from build123d import *

# Parameters (mm, degrees)
BOSS_EXTRUDE1_DEPTH = 534.6
SKETCH2_R           = 12.7
CUT_EXTRUDE1_DEPTH  = 18.288
SKETCH3_R           = 14
CUT_EXTRUDE2_DEPTH  = 18.288
SKETCH4_R           = 14
CUT_EXTRUDE3_DEPTH  = 18.288


with BuildPart() as part:
    # Sketch1 → Boss-Extrude1 (new body)
    with BuildSketch(Plane.XY):
        Polygon((0, 0), (5.762672042, 402.6498479), (18.424747765, 400), (12.7, 0), align=None)
    extrude(amount=BOSS_EXTRUDE1_DEPTH)

    # Sketch2 → Cut-Extrude1 (cut)
    with BuildSketch(Plane(origin=(12.697399197, -0.181723519, 0), x_dir=(0, 0, -1), z_dir=(0.9998976009274501, -0.014310403891230014, 0))):
        with Locations(Location((-88.9, 254.181742129, 0), (0, 0, 90))):
            Circle(SKETCH2_R)
    extrude(amount=-CUT_EXTRUDE1_DEPTH, mode=Mode.SUBTRACT)

    # Sketch3 → Cut-Extrude2 (cut)
    with BuildSketch(Plane(origin=(12.697399197, -0.181723519, 0), x_dir=(0, 0, -1), z_dir=(0.9998976009274501, -0.014310403891230014, 0))):
        with Locations(Location((-88.9, 127.181742129, 0), (0, 0, 90))):
            Circle(SKETCH3_R)
    extrude(amount=-CUT_EXTRUDE2_DEPTH, mode=Mode.SUBTRACT)

    # Sketch4 → Cut-Extrude3 (cut)
    with BuildSketch(Plane(origin=(12.697399197, -0.181723519, 0), x_dir=(0, 0, -1), z_dir=(0.9998976009274501, -0.014310403891230014, 0))):
        with Locations(Location((-445.7, 254.181742129, 0), (0, 0, 90))):
            Circle(SKETCH4_R)
    extrude(amount=-CUT_EXTRUDE3_DEPTH, mode=Mode.SUBTRACT)


solid = part.part
Model file for the job. Use its own axes, mm. Give positions to 0.01 mm unless a question says otherwise; leave off trailing zeros. Order: outer loops, then holes, each group sorted by start corner. A loop starts at its lowest first (then second) coordinate and runs counter-clockwise, first axis right, second up. Notation, with made-up numbers: (46, 65.25) - (62, 65.25) arc R25 cw to (62, 85.25) - close; hole circle Ø3 at (85.25, 69.5). An arc over 180 degrees is marked (long way). Write item = value, one per line. Start each with the question number.
1. Cut at A-A, the plane z = 336. List the corners of the cut face in (x, y), and give its area (3 significant figures).
2. Probe line 1 along Z through (x, y) = (14.25, 253); line 2 along Z through (x, y) = (9.75, 264); line 3 along Y through (x, z) = (10, 86). List the from-to ranges inside material, lowest first.
3. Two-plate mould, pull along Y, no slides. Class faces 1 (the flat face through (6, 0, 264)), 2 (the cylindrical face through (8.23, 125.25, 102.78)), 3 (the flat face through (9, 204, 534.6)): pulls with the +Y half, pulls with the -Y half, needs draft (parallel to the pull), parting line crosses it, or undercut.
4. Cut at B-B, the plane y = 247.5. State how many separate pieces and enclosed holes the cut face has, and give its area (3 significant figures).
5. Drop flat-ended pins along their axis: P1, Ø10, axis at y = 174, z = 218.5, coming from the -X side; P2, Ø4, axis at y = 113.5, z = 317, coming from the -X side; P3, Ø2, axis at x = 9, z = 232.5, coming from the +Y side. Give the stop position or say it passes through.
Taken from the geometry:
q1.outline = (0, 0) - (12.7, 0) - (18.42, 400) - (5.76, 402.65) - close
q1.area = 5,100 mm²
q2.line_1 = 0 to 76.24, 101.56 to 431.74, 459.66 to 534.6
q2.line_2 = 0 to 80.98, 96.82 to 435.83, 455.57 to 534.6
q2.line_3 = 0 to 113.35, 140.75 to 241.7, 266.43 to 401.76
q3.face_1 = pulls with the -Y half
q3.face_2 = undercut
q3.face_3 = needs draft
q4.separate_pieces = 3
q4.enclosed_holes = 0
q4.area = 6,200 mm²
q5.P1 = 2.42
q5.P2 = 1.6
q5.P3 = 402.18
